Drawing for the job (mm, zero at the part's lowest x, y, z). A direction names the side the tool comes from. Round coordinates to 2 decimals unless told otherwise and drop trailing zeros. Write each loop counter-clockwise with the first axis right and the second up, starting at its lowest first coordinate (ties: lowest second). Pieces come first, ordered by that corner, then holes. Notation, with made-up numbers: M 50,59.25 L 62,59.25 A12 cw 62,78.25 Z; hole C 63,3 d7. An arc over 180 degrees is marked long. Use a Markdown table: item, result. Add a question column.
1) Drop flat-ended pins along their axis: P1, Ø20.5, axis at x = 51.5, z = 36, coming from the +Y side; P2, Ø8, axis at y = 36.5, z = 44.5, coming from the -X side; P3, Ø5.5, axis at x = 18.5, y = 27.5, coming from the +Z side; P4, Ø8, axis at x = 97, y = 52, coming from the -Z side. Give the stop position or say it passes through.
2) Which spindle directions (+Z, -Z, +X, -X, +Y, -Y) get a long thin tool onto all of the face, cutting with end or side? Do the marked faces 1, 2 and 3. Say none if no direction does.
3) Slice it at C-C on y = 19. Write the cut outline in (x, z).
4) Slice it at D-D on z = 43.5. Write the cut outline in (x, y).
5) Slice it at A-A on z = 30. Write the cut outline in (x, y), plus the area to 3 significant figures.
6) Two-plate mould, pull along Y, no slides. Class the marked faces 4, 5 and 6: released by +Y, released by -Y, zero draft, split by the parting line, or undercut.
7) Wall check: probe 1 along Y at (x, z) = (6, 27.5); probe 2 along X at (y, z) = (31, 16); probe 3 along Y at (x, z) = (83.5, 34.5). Give the ranges that are in metal, low to high.
8) Slice it at B-B on x = 26.5. Write the cut outline in (y, z), plus the area to 3 significant figures.
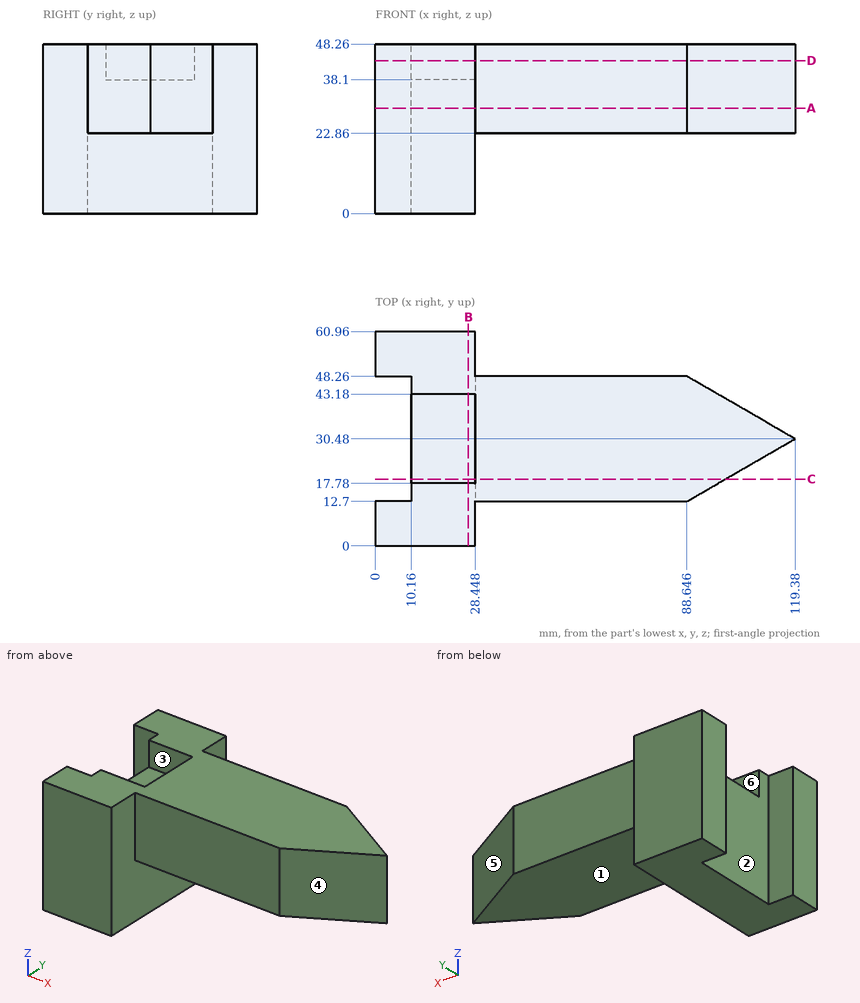
Entries:
| question | item | result |
|---|---|---|
| 1 | P1 | stops at y = 48.26 |
| 1 | P2 | stops at x = 28.45 |
| 1 | P3 | stops at z = 38.1 |
| 1 | P4 | passes through |
| 2 | face 1 | -Z, +X, +Y, -Y |
| 2 | face 2 | +Z, -Z, -X |
| 2 | face 3 | +Z, -X |
| 3 | outline | M 10.16,0 L 28.45,0 L 28.45,22.86 L 99.54,22.86 L 99.54,48.26 L 28.45,48.26 L 28.45,38.1 L 10.16,38.1 Z |
| 4 | outline | M 0,0 L 28.45,0 L 28.45,12.7 L 88.65,12.7 L 119.38,30.48 L 88.65,48.26 L 28.45,48.26 L 28.45,60.96 L 0,60.96 L 0,48.26 L 10.16,48.26 L 10.16,43.18 L 28.45,43.18 L 28.45,17.78 L 10.16,17.78 L 10.16,12.7 L 0,12.7 Z |
| 5 | outline | M 0,0 L 28.45,0 L 28.45,12.7 L 88.65,12.7 L 119.38,30.48 L 88.65,48.26 L 28.45,48.26 L 28.45,60.96 L 0,60.96 L 0,48.26 L 10.16,48.26 L 10.16,12.7 L 0,12.7 Z |
| 5 | area | 4,060 mm^2 |
| 6 | face 4 | released by -Y |
| 6 | face 5 | released by +Y |
| 6 | face 6 | undercut |
| 7 | probe 1 | y = 0 to 12.7, 48.26 to 60.96 |
| 7 | probe 2 | x = 10.16 to 28.45 |
| 7 | probe 3 | y = 12.7 to 48.26 |
| 8 | outline | M 0,0 L 60.96,0 L 60.96,48.26 L 43.18,48.26 L 43.18,38.1 L 17.78,38.1 L 17.78,48.26 L 0,48.26 Z |
| 8 | area | 2,680 mm^2 |
